Check sheet for the modelled part. Datum: model origin and axes. Units: mm. A direction names the side the tool comes from. Round coordinates to 2 decimals unless told otherwise and drop trailing zeros. Write each loop counter-clockwise with the first axis right and the second up, starting at its lowest first coordinate (ties: lowest second). Pieces come first, ordered by that corner, then holes. Notation, with made-up numbers: (-19, 7) - (32, 7) arc R8 cw to (32, 15) - close; hole circle Ø5 at (82.5, 69.25). An arc over 180 degrees is marked (long way). Use one line per item in the form item = value. Start each with the question number.
1) Set-up check for faces 1 (the face through (-31.52, -12.52, 11.87)), 2 (the face through (16.13, -12.52, -56.2)), 3 (the face through (-26.071, -12.522, 21.227)), 4 (the face through (41.144, -12.522, -32.431)), 5 (the face through (32.267, -12.522, -32.453)): record each of +Z, -Z, +X, -X, +Y, -Y from which the full face is reachable in a straight line by a thin tool's end or side.
2) Draft check along X on faces 6 (the face through (-15.952, -12.522, -27.451)), 7 (the face through (-48.658, -12.522, -19.416)), 8 (the face through (-1, -25.4, 1)). Enter one of: +X half, -X half, draft (parallel to the pull), parting line (faces both ways), or undercut.
3) Gauge pin test, flat ends, axial feed: P1, Ø1.2, axis at y = -12, z = 33, coming from the +X side; P2, Ø4.5, axis at y = -13.5, z = -32.5, coming from the +X side; P3, Ø6, axis at x = -40, z = -25, coming from the -Y side; P4, Ø5, axis at y = -19.5, z = 18, coming from the +X side. Record the tip position at first contact, or that the pin passes through.
4) Scan lines: probe 1 along X at (y, z) = (-22.5, -22.5); probe 2 along Z at (x, y) = (-16, -18.5); probe 3 along Z at (x, y) = (40, -9.5). Record each from-to range of solid material in increasing order.
5) Section check B-B (x = 23). Record the boundary of the cut face in (y, z).
6) Section check A-A (z = -5). Record the boundary of the cut face in (x, y), then the cut area to 3 significant figures.
from build123d import *

# Parameters (mm, degrees)
F1_DEPTH = 25.4


# Not quite as in the source:
# - a feature names something its author has since deleted; it is built from what else it names


with BuildPart() as f1:
    # F0 (on Front) → F1 (new body)
    with BuildSketch(Plane.XZ):
        with BuildLine():
            ThreePointArc((29.8236565437, -10.8909141198), (31.2647053022, -5.529982131), (31.75, 0))
            ThreePointArc((31.75, 0), (31.2529370271, 5.5961082175), (29.7773116736, 11.0169963917))
            ThreePointArc((29.7773116736, 11.0169963917), (27.4626625114, 15.9331311356), (24.34363657, 20.3825871407))
            ThreePointArc((24.34363657, 20.3825871407), (15.8167978227, 27.529827581), (5.3476570882, 31.2964065616))
            ThreePointArc((5.3476570882, 31.2964065616), (-0.0671650695, 31.7499289582), (-5.4800199737, 31.2735012605))
            ThreePointArc((-5.4800199737, 31.2735012605), (-15.9331311356, 27.4626625114), (-24.4296545854, 20.2794101699))
            ThreePointArc((-24.4296545854, 20.2794101699), (-27.529827581, 15.8167978227), (-29.8236565437, 10.8909141198))
            ThreePointArc((-29.8236565437, 10.8909141198), (-31.7499289582, -0.0671650695), (-29.7773116736, -11.0169963917))
            ThreePointArc((-29.7773116736, -11.0169963917), (-27.4626625114, -15.9331311356), (-24.34363657, -20.3825871407))
            ThreePointArc((-24.34363657, -20.3825871407), (-15.8167978227, -27.529827581), (-5.3476570882, -31.2964065616))
            ThreePointArc((-5.3476570882, -31.2964065616), (0.0671650695, -31.7499289582), (5.4800199737, -31.2735012605))
            ThreePointArc((5.4800199737, -31.2735012605), (15.9331311356, -27.4626625114), (24.4296545854, -20.2794101699))
            ThreePointArc((24.4296545854, -20.2794101699), (27.529827581, -15.8167978227), (29.8236565437, -10.8909141198))
        make_face()
        with BuildLine():
            ThreePointArc((-29.8236565437, 10.8909141198), (-27.529827581, 15.8167978227), (-24.4296545854, 20.2794101699))
            Line((-24.4296545854, 20.2794101699), (-27.7596928163, 22.2020086389))
            ThreePointArc((-27.7596928163, 22.2020086389), (-28.0803819304, 22.4654648728), (-28.2990076095, 22.8182445595))
            Line((-28.2990076095, 22.8182445595), (-36.3474772559, 42.3614984651))
            ThreePointArc((-36.3474772559, 42.3614984651), (-37.0333944907, 43.0502164715), (-38.0054083913, 43.0521969161))
            Line((-38.0054083913, 43.0521969161), (-43.2545602789, 40.8904463786))
            ThreePointArc((-43.2545602789, 40.8904463786), (-43.9432782853, 40.2045291438), (-43.9452587299, 39.2325152431))
            Line((-43.9452587299, 39.2325152431), (-38.2633402939, 25.4357091987))
            ThreePointArc((-38.2633402939, 25.4357091987), (-38.17045953, 24.8677399071), (-38.3378028243, 24.3170928565))
            Line((-38.3378028243, 24.3170928565), (-39.3160529196, 22.622713989))
            Line((-39.3160529196, 22.622713989), (-40.2943030148, 20.9283351216))
            ThreePointArc((-40.2943030148, 20.9283351216), (-40.687505702, 20.5080880523), (-41.225821919, 20.3045405075))
            Line((-41.225821919, 20.3045405075), (-56.0151656626, 18.3268231931))
            ThreePointArc((-56.0151656626, 18.3268231931), (-56.8559641711, 17.8391011274), (-57.1056269181, 16.8996952205))
            Line((-57.1056269181, 16.8996952205), (-56.3531818565, 11.2729210687))
            ThreePointArc((-56.3531818565, 11.2729210687), (-55.8654597908, 10.4321225602), (-54.9260538839, 10.1824598132))
            Line((-54.9260538839, 10.1824598132), (-33.9768647058, 12.9839075907))
            ThreePointArc((-33.9768647058, 12.9839075907), (-33.5620356955, 12.970962042), (-33.1735313472, 12.8249652394))
            Line((-33.1735313472, 12.8249652394), (-29.8236565437, 10.8909141198))
        make_face()
        with BuildLine():
            ThreePointArc((-5.4800199737, 31.2735012605), (-0.0671650695, 31.7499289582), (5.3476570882, 31.2964065616))
            Line((5.3476570882, 31.2964065616), (5.3476570882, 35.1416034996))
            ThreePointArc((5.3476570882, 35.1416034996), (5.4154723224, 35.551056536), (5.6116756536, 35.9167817715))
            Line((5.6116756536, 35.9167817715), (18.5123951852, 52.6585878997))
            ThreePointArc((18.5123951852, 52.6585878997), (18.7658838574, 53.596968653), (18.2815920225, 54.4397476062))
            Line((18.2815920225, 54.4397476062), (13.7848851965, 57.9047712204))
            ThreePointArc((13.7848851965, 57.9047712204), (12.8465044431, 58.1582598926), (12.00372549, 57.6739680576))
            Line((12.00372549, 57.6739680576), (2.8963001824, 45.8548793275))
            ThreePointArc((2.8963001824, 45.8548793275), (2.4508647292, 45.4904575807), (1.8903187477, 45.3600575994))
            Line((1.8903187477, 45.3600575994), (-0.0661814427, 45.3600575994))
            Line((-0.0661814427, 45.3600575994), (-2.0226816332, 45.3600575994))
            ThreePointArc((-2.0226816332, 45.3600575994), (-2.5832276147, 45.4904575807), (-3.0286630678, 45.8548793275))
            Line((-3.0286630678, 45.8548793275), (-12.1360883754, 57.6739680576))
            ThreePointArc((-12.1360883754, 57.6739680576), (-12.9788673285, 58.1582598926), (-13.9172480819, 57.9047712204))
            Line((-13.9172480819, 57.9047712204), (-18.4139549079, 54.4397476062))
            ThreePointArc((-18.4139549079, 54.4397476062), (-18.8982467429, 53.596968653), (-18.6447580707, 52.6585878997))
            Line((-18.6447580707, 52.6585878997), (-5.744038539, 35.9167817715))
            ThreePointArc((-5.744038539, 35.9167817715), (-5.5478352079, 35.551056536), (-5.4800199737, 35.1416034996))
            Line((-5.4800199737, 35.1416034996), (-5.4800199737, 31.2735012605))
        make_face()
        with BuildLine():
            ThreePointArc((24.34363657, 20.3825871407), (27.4626625114, 15.9331311356), (29.7773116736, 11.0169963917))
            Line((29.7773116736, 11.0169963917), (33.1073499045, 12.9395948607))
            ThreePointArc((33.1073499045, 12.9395948607), (33.4958542528, 13.0855916633), (33.9106832631, 13.098537212))
            Line((33.9106832631, 13.098537212), (54.8598724411, 10.2970894345))
            ThreePointArc((54.8598724411, 10.2970894345), (55.7992783481, 10.5467521815), (56.2870004138, 11.38755069))
            Line((56.2870004138, 11.38755069), (57.0394454754, 17.0143248418))
            ThreePointArc((57.0394454754, 17.0143248418), (56.7897827284, 17.9537307487), (55.9489842199, 18.4414528144))
            Line((55.9489842199, 18.4414528144), (41.1596404763, 20.4191701289))
            ThreePointArc((41.1596404763, 20.4191701289), (40.6213242593, 20.6227176736), (40.2281215721, 21.0429647429))
            Line((40.2281215721, 21.0429647429), (39.2498714768, 22.7373436104))
            Line((39.2498714768, 22.7373436104), (38.2716213816, 24.4317224778))
            ThreePointArc((38.2716213816, 24.4317224778), (38.1042780873, 24.9823695284), (38.1971588512, 25.55033882))
            Line((38.1971588512, 25.55033882), (43.8790772872, 39.3471448645))
            ThreePointArc((43.8790772872, 39.3471448645), (43.8770968426, 40.3191587651), (43.1883788362, 41.0050759999))
            Line((43.1883788362, 41.0050759999), (37.9392269486, 43.1668265375))
            ThreePointArc((37.9392269486, 43.1668265375), (36.9672130479, 43.1648460928), (36.2812958132, 42.4761280865))
            Line((36.2812958132, 42.4761280865), (28.2328261668, 22.9328741809))
            ThreePointArc((28.2328261668, 22.9328741809), (28.0142004876, 22.5800944941), (27.6935113736, 22.3166382603))
            Line((27.6935113736, 22.3166382603), (24.34363657, 20.3825871407))
        make_face()
        with BuildLine():
            Line((33.1735313472, -12.8249652394), (29.8236565437, -10.8909141198))
            ThreePointArc((29.8236565437, -10.8909141198), (27.529827581, -15.8167978227), (24.4296545854, -20.2794101699))
            Line((24.4296545854, -20.2794101699), (27.7596928163, -22.2020086389))
            ThreePointArc((27.7596928163, -22.2020086389), (28.0803819304, -22.4654648728), (28.2990076095, -22.8182445595))
            Line((28.2990076095, -22.8182445595), (36.3474772559, -42.3614984651))
            ThreePointArc((36.3474772559, -42.3614984651), (37.0333944907, -43.0502164715), (38.0054083913, -43.0521969161))
            Line((38.0054083913, -43.0521969161), (43.2545602789, -40.8904463786))
            ThreePointArc((43.2545602789, -40.8904463786), (43.9432782853, -40.2045291438), (43.9452587299, -39.2325152431))
            Line((43.9452587299, -39.2325152431), (38.2633402939, -25.4357091987))
            ThreePointArc((38.2633402939, -25.4357091987), (38.17045953, -24.8677399071), (38.3378028243, -24.3170928565))
            Line((38.3378028243, -24.3170928565), (39.3160529196, -22.622713989))
            Line((39.3160529196, -22.622713989), (40.2943030148, -20.9283351216))
            ThreePointArc((40.2943030148, -20.9283351216), (40.687505702, -20.5080880523), (41.225821919, -20.3045405075))
            Line((41.225821919, -20.3045405075), (56.0151656626, -18.3268231931))
            ThreePointArc((56.0151656626, -18.3268231931), (56.8559641711, -17.8391011274), (57.1056269181, -16.8996952205))
            Line((57.1056269181, -16.8996952205), (56.3531818565, -11.2729210687))
            ThreePointArc((56.3531818565, -11.2729210687), (55.8654597908, -10.4321225602), (54.9260538839, -10.1824598132))
            Line((54.9260538839, -10.1824598132), (33.9768647058, -12.9839075907))
            ThreePointArc((33.9768647058, -12.9839075907), (33.5620356955, -12.970962042), (33.1735313472, -12.8249652394))
        make_face()
        with BuildLine():
            Line((5.4800199737, -35.1416034996), (5.4800199737, -31.2735012605))
            ThreePointArc((5.4800199737, -31.2735012605), (0.0671650695, -31.7499289582), (-5.3476570882, -31.2964065616))
            Line((-5.3476570882, -31.2964065616), (-5.3476570882, -35.1416034996))
            ThreePointArc((-5.3476570882, -35.1416034996), (-5.4154723224, -35.551056536), (-5.6116756536, -35.9167817715))
            Line((-5.6116756536, -35.9167817715), (-18.5123951852, -52.6585878997))
            ThreePointArc((-18.5123951852, -52.6585878997), (-18.7658838574, -53.596968653), (-18.2815920225, -54.4397476062))
            Line((-18.2815920225, -54.4397476062), (-13.7848851965, -57.9047712204))
            ThreePointArc((-13.7848851965, -57.9047712204), (-12.8465044431, -58.1582598926), (-12.00372549, -57.6739680576))
            Line((-12.00372549, -57.6739680576), (-2.8963001824, -45.8548793275))
            ThreePointArc((-2.8963001824, -45.8548793275), (-2.4508647292, -45.4904575807), (-1.8903187477, -45.3600575994))
            Line((-1.8903187477, -45.3600575994), (0.0661814427, -45.3600575994))
            Line((0.0661814427, -45.3600575994), (2.0226816332, -45.3600575994))
            ThreePointArc((2.0226816332, -45.3600575994), (2.5832276147, -45.4904575807), (3.0286630678, -45.8548793275))
            Line((3.0286630678, -45.8548793275), (12.1360883754, -57.6739680576))
            ThreePointArc((12.1360883754, -57.6739680576), (12.9788673285, -58.1582598926), (13.9172480819, -57.9047712204))
            Line((13.9172480819, -57.9047712204), (18.4139549079, -54.4397476062))
            ThreePointArc((18.4139549079, -54.4397476062), (18.8982467429, -53.596968653), (18.6447580707, -52.6585878997))
            Line((18.6447580707, -52.6585878997), (5.744038539, -35.9167817715))
            ThreePointArc((5.744038539, -35.9167817715), (5.5478352079, -35.551056536), (5.4800199737, -35.1416034996))
        make_face()
        with BuildLine():
            Line((-27.6935113736, -22.3166382603), (-24.34363657, -20.3825871407))
            ThreePointArc((-24.34363657, -20.3825871407), (-27.4626625114, -15.9331311356), (-29.7773116736, -11.0169963917))
            Line((-29.7773116736, -11.0169963917), (-33.1073499045, -12.9395948607))
            ThreePointArc((-33.1073499045, -12.9395948607), (-33.4958542528, -13.0855916633), (-33.9106832631, -13.098537212))
            Line((-33.9106832631, -13.098537212), (-54.8598724411, -10.2970894345))
            ThreePointArc((-54.8598724411, -10.2970894345), (-55.7992783481, -10.5467521815), (-56.2870004138, -11.38755069))
            Line((-56.2870004138, -11.38755069), (-57.0394454754, -17.0143248418))
            ThreePointArc((-57.0394454754, -17.0143248418), (-56.7897827284, -17.9537307487), (-55.9489842199, -18.4414528144))
            Line((-55.9489842199, -18.4414528144), (-41.1596404763, -20.4191701289))
            ThreePointArc((-41.1596404763, -20.4191701289), (-40.6213242593, -20.6227176736), (-40.2281215721, -21.0429647429))
            Line((-40.2281215721, -21.0429647429), (-39.2498714768, -22.7373436104))
            Line((-39.2498714768, -22.7373436104), (-38.2716213816, -24.4317224778))
            ThreePointArc((-38.2716213816, -24.4317224778), (-38.1042780873, -24.9823695284), (-38.1971588512, -25.55033882))
            Line((-38.1971588512, -25.55033882), (-43.8790772872, -39.3471448645))
            ThreePointArc((-43.8790772872, -39.3471448645), (-43.8770968426, -40.3191587651), (-43.1883788362, -41.0050759999))
            Line((-43.1883788362, -41.0050759999), (-37.9392269486, -43.1668265375))
            ThreePointArc((-37.9392269486, -43.1668265375), (-36.9672130479, -43.1648460928), (-36.2812958132, -42.4761280865))
            Line((-36.2812958132, -42.4761280865), (-28.2328261668, -22.9328741809))
            ThreePointArc((-28.2328261668, -22.9328741809), (-28.0142004876, -22.5800944941), (-27.6935113736, -22.3166382603))
        make_face()
    extrude(amount=F1_DEPTH)


solid = f1.part
Results are:
q1.face_1 = +Y, -Y
q1.face_2 = -Z, +X, +Y, -Y
q1.face_3 = +Z, +Y, -Y
q1.face_4 = +X, +Y, -Y
q1.face_5 = -Z, +Y, -Y
q2.face_6 = undercut
q2.face_7 = -X half
q2.face_8 = draft
q3.P1 = 41.51
q3.P2 = 42.1
q3.P3 = -25.4
q3.P4 = 57.05
q4.probe_1 = -39.39 to -27.94, -22.4 to 22.4, 28.11 to 39.39
q4.probe_2 = -56.2 to -49.4, -27.42 to 27.42, 49.23 to 56.3
q4.probe_3 = -42.23 to -29.65, -21.44 to -12.18, 12.28 to 21.44, 29.93 to 42.32
q5.outline = (-25.4, -21.89) - (0, -21.89) - (0, 21.89) - (-25.4, 21.89) - close
q6.outline = (-31.35, -25.4) - (31.35, -25.4) - (31.35, 0) - (-31.35, 0) - close
q6.area = 1,590 mm²
